Can you work these out from the model? Positions are in its coordinate system, mm. Face numbers are marked on the shaded views. A direction names the side the tool comes from. Round coordinates to 2 decimals unless told otherwise and drop trailing zeros. Write each loop counter-clockwise with the first axis right and the second up, starting at its lowest first coordinate (ties: lowest second). Pieces come first, ordered by that corner, then holes. Notation, with made-up numbers: M -3.5,87.5 L 52.5,87.5 A15 cw 52.5,116.5 Z; hole C 32.5,-8 d7. An arc over 180 degrees is marked long. Use one line per item in the form item = value. Start each with the question number.
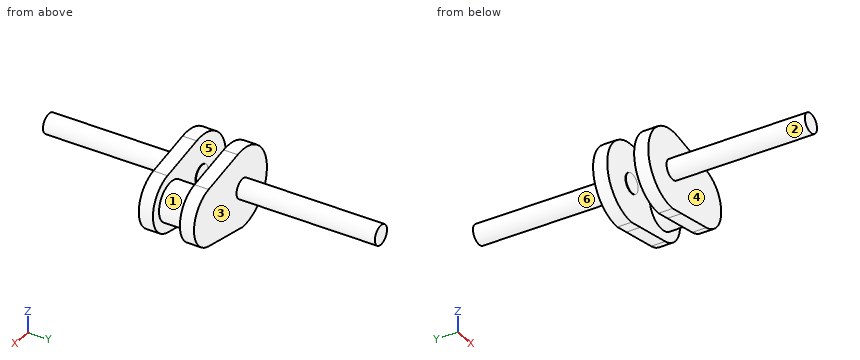
```python
from build123d import *

# Parameters (mm, degrees)
F0_R     = 5.08
F0_R_2   = 10.16
F1_DEPTH = 7.366
F2_R     = 10.16
F3_DEPTH = 6.99897
F7_R     = 5.08
F8_DEPTH = 79.5782


# Not quite as in the source:
# - a length typed as a fraction of an inch, garbled in the dataset ("3 / 203.2 mm" for 3/8 in), is restored


with BuildPart() as f1:
    # F0 (on Front) → F1 (new body)
    with BuildSketch(Plane.XZ):
        with BuildLine():
            Line((28.448, 14.932089472), (4.064, 19.9094526293))
            ThreePointArc((4.064, 19.9094526293), (-20.2171026291, 2.0423421079), (0, -20.32))
            Line((0, -20.32), (7.4284633963, -18.9134960166))
            Line((7.4284633963, -18.9134960166), (28.2351667085, -14.9739583856))
            ThreePointArc((28.2351667085, -14.9739583856), (40.639614078, -0.1084562307), (28.448, 14.932089472))
        make_face()
        Circle(F0_R, mode=Mode.SUBTRACT)
        with Locations((25.4, 0)):
            Circle(F0_R_2, mode=Mode.SUBTRACT)
        with Locations((25.4, 0)):
            Circle(F0_R_2)
    extrude(amount=F1_DEPTH)

    # F2 (on face) → F3 (join)
    with BuildSketch(Plane.XZ.offset(7.366)):
        with Locations((25.4, 0)):
            Circle(F2_R)
    extrude(amount=F3_DEPTH)

    # F5: F1 across plane


with BuildPart() as f1_1:
    add(f1.part)
    add(f1.part.mirror(Plane(origin=(25.4, -14.36497, 0), x_dir=(1, 0, 0), z_dir=(0, -1, 0))))

    # F7 (on offset) → F8 (join)
    with BuildSketch(Plane.XZ.offset(21.10994)):
        Circle(F7_R)
    extrude(amount=F8_DEPTH)

    # F9: F1 across plane


with BuildPart() as f1_2:
    add(f1_1.part)
    add(f1_1.part.mirror(Plane(origin=(25.4, -14.36497, 0), x_dir=(1, 0, 0), z_dir=(0, -1, 0))))


solid = f1_2.part
```
1. If we section it at B-B (y = 39): List the corners of the cut face in (x, z) for me.
2. If we section it at D-D (x = 17): List the corners of the cut face in (y, z) for me.
3. If we mould it in two halves opening along Y, with no side actions, what happens to the marked faces 4, 5 and 6? For each: pulls with the +Y half, pulls with the -Y half, needs draft (parallel to the pull), parting line crosses it, or undercut.
4. Which directions (+Z, -Z, +X, -X, +Y, -Y) give clear straight access to the entire face, cutting with the end or side of a thin tool? Please do the marked faces 1, 2 and 3.
5. Will these pins go through, and if not, where does the flat tip stop? pin 1 (1 mm diameter, centred on y = -19.5, z = -5.5, fed in from +X); pin 2 (1.5 mm diameter, centred on y = -45.5, z = 0, fed in from -X); pin 3 (6 mm diameter, centred on x = -9, z = 7.5, fed in from +Y).
6. If we section it at A-A (z = 0): List the corners of the cut face in (x, y) for me.
7. Please list where these lines run through material, in increasing order: line 1 along Y through (x, z) = (27.5, 10.5); line 2 along Y through (x, z) = (18, -2.5); line 3 along X through (y, z) = (16, 4.5).
8. If we section it at C-C (x = 32): List the corners of the cut face in (y, z) for me.
Model answer:
q1.outline = C 0,0 d10.16
q2.outline = M -28.73,-17.1 L -21.36,-17.1 L -21.36,-5.72 L -7.37,-5.72 L -7.37,-17.1 L 0,-17.1 L 0,17.27 L -7.37,17.27 L -7.37,5.72 L -21.36,5.72 L -21.36,17.27 L -28.73,17.27 Z
q3.face_4 = pulls with the -Y half
q3.face_5 = undercut
q3.face_6 = needs draft
q4.face_1 = none
q4.face_2 = -Y
q4.face_3 = +Y
q5.pin_1 = 34.24
q5.pin_2 = -5.08
q5.pin_3 = 0
q6.outline = M -20.32,-28.73 L -5.08,-28.73 L -5.08,-100.69 L 5.08,-100.69 L 5.08,-28.73 L 40.64,-28.73 L 40.64,-21.36 L 35.56,-21.36 L 35.56,-7.37 L 40.64,-7.37 L 40.64,0 L 5.08,0 L 5.08,71.96 L -5.08,71.96 L -5.08,0 L -20.32,0 L -20.32,-7.37 L -5.08,-7.37 L -5.08,-7.62 L 5.08,-7.62 L 5.08,-7.37 L 15.24,-7.37 L 15.24,-21.36 L 5.08,-21.36 L 5.08,-21.11 L -5.08,-21.11 L -5.08,-21.36 L -20.32,-21.36 Z
q7.line_1 = -28.73 to -21.36, -7.37 to 0
q7.line_2 = -28.73 to 0
q7.line_3 = -2.36 to 2.36
q8.outline = M -28.73,-13.74 L -21.36,-13.74 L -21.36,-7.72 L -7.37,-7.72 L -7.37,-13.74 L 0,-13.74 L 0,13.74 L -7.37,13.74 L -7.37,7.72 L -21.36,7.72 L -21.36,13.74 L -28.73,13.74 Z
